from build123d import *

# Parameters (mm, degrees)
SKETCH2_W           = 16.5
SKETCH2_H           = 15.758588826
BOSS_EXTRUDE1_DEPTH = 3
SKETCH3_W           = 16.5
SKETCH3_H           = 4.058588826
BOSS_EXTRUDE2_DEPTH = 1.4
SKETCH4_W           = 16.5
SKETCH4_H           = 10.7
SKETCH4_R           = 1.65
BOSS_EXTRUDE3_DEPTH = 3
SKETCH5_R           = 1.4
CUT_EXTRUDE1_DEPTH  = 3
CHAMFER1_SIZE       = 2
SKETCH6_R           = 4.45
CUT_EXTRUDE2_DEPTH  = 17


with BuildPart() as part:
    # Sketch2 → Boss-Extrude1 (new body)
    with BuildSketch(Plane.XY):
        with Locations((0, 3.620705587)):
            Rectangle(SKETCH2_W, SKETCH2_H)
    extrude(amount=BOSS_EXTRUDE1_DEPTH)

    # Sketch3 → Boss-Extrude2 (add)
    with BuildSketch(Plane(origin=(0, 0, 0), x_dir=(-1, 0, 0), z_dir=(0, 0, -1))):
        with Locations((0, -2.229294413)):
            Rectangle(SKETCH3_W, SKETCH3_H)
    extrude(amount=BOSS_EXTRUDE2_DEPTH)

    # Sketch4 → Boss-Extrude3 (add)
    with BuildSketch(Plane(origin=(0, 0, -1.4), x_dir=(-1, 0, 0), z_dir=(0, 0, -1))):
        with Locations((0, -5.55)):
            Rectangle(SKETCH4_W, SKETCH4_H)
        with Locations((-5.25, -7.2)):
            Circle(SKETCH4_R, mode=Mode.SUBTRACT)
        with Locations((5.25, -7.2)):
            Circle(SKETCH4_R, mode=Mode.SUBTRACT)
    extrude(amount=BOSS_EXTRUDE3_DEPTH)

    # Sketch5 → Cut-Extrude1 (cut)
    with BuildSketch(Plane(origin=(0, 0, 0), x_dir=(-1, 0, 0), z_dir=(0, 0, -1))):
        with Locations((-5.25, 3.5)):
            Circle(SKETCH5_R)
        with Locations((5.25, 3.5)):
            Circle(SKETCH5_R)
    extrude(amount=-CUT_EXTRUDE1_DEPTH, mode=Mode.SUBTRACT)

    # Chamfer1
    chamfer1_edges = [part.edges().sort_by_distance(p)[0] for p in [
        (8.25, -10.9, -2.9),
        (-8.25, -10.9, -2.9),
        (-8.25, 11.5, 1.5),
        (8.25, 11.5, 1.5),
    ]]
    chamfer(chamfer1_edges, length=CHAMFER1_SIZE)

    # Sketch6 → Cut-Extrude2 (cut)
    with BuildSketch(Plane(origin=(0, -0.2, 0), x_dir=(1, 0, 0), z_dir=(0, 1, 0))):
        with Locations((0, 8.5)):
            Circle(SKETCH6_R)
    extrude(amount=-CUT_EXTRUDE2_DEPTH, mode=Mode.SUBTRACT)


solid = part.part
Work out the finished part from the listing and answer in its coordinate system (mm). A direction names the side the tool comes from. Give positions to 0.01 mm unless a question says otherwise; leave off trailing zeros. Loops run counter-clockwise (first coordinate to the right, second up) from the corner with the lowest first, then second, coordinate; pieces in that order, holes last. Notation, with made-up numbers: (35.25, -13) -> (66.25, -13) arc R24 ccw to (66.25, 26) -> close; hole circle Ø2 at (58, 89). An arc over 180 degrees is marked (long way). Use a Markdown table: item, result. Add a question column.
1) Which of the six approach directions +Z, -Z, +X, -X, +Y, -Y give full straight-line access (tool end or side, diameter ignored) to faces 1 (the flat face through (0, 6, 0)), 2 (the cylindrical face through (-4.034, -6.085, -2.879)), 3 (the flat face through (0, -4.259, 1))?
2) Consider line 1 along Y through (x, z) = (-5.25, 1.6); line 2 along X through (y, z) = (4.75, 1); line 3 along Y through (x, z) = (-5.25, -2.25). Determine where each line is inside the solid, lowest interval first.
3) The part is cut by section B-B, the plane z = -2.5. Determine the outline of the cut face in (x, y), plus the area to 3 significant figures.
4) The part is cut by section D-D, the plane x = -3. Determine the outline of the cut face in (y, z).
5) The part is cut by section C-C, the plane x = -5.25. Determine the outline of the cut face in (y, z), plus the area to 3 significant figures.
6) The part is cut by section A-A, the plane y = 3.5. Determine the outline of the cut face in (x, z).
7) Each of these flat-tipped pins is pushed along its axis until it touches: P1, Ø2, axis at x = -3.5, y = -7.5, coming from the +Z side; P2, Ø1, axis at x = 5, y = 6.5, coming from the -Z side; P3, Ø2, axis at x = -3.5, z = -3, coming from the +Y side. Where does it stop, or does it pass through?
8) For a pull along Y with two mould halves and no side action, classify faces 4 (the flat face through (-8.25, 0.2, 0.2)), 5 (the flat face through (0, 11.5, 1)), 6 (the cylindrical face through (-5.9, 2.26, 1.48)) as +Y half, -Y half, draft (parallel to the pull), parting line (faces both ways), or undercut.
Reported:
| question | item | result |
|---|---|---|
| 1 | face 1 | -Z, +X, -X, +Y |
| 1 | face 2 | +Z, -Z |
| 1 | face 3 | +Z, +X, -X, -Y |
| 2 | line 1 | y = -4.26 to 2.1, 4.9 to 11.5 |
| 2 | line 2 | x = -8.25 to -5.88, -4.62 to 4.62, 5.88 to 8.25 |
| 2 | line 3 | y = -10.9 to -8.85, -5.55 to -0.2 |
| 3 | outline | (-8.25, -8.9) -> (-6.25, -10.9) -> (6.25, -10.9) -> (8.25, -8.9) -> (8.25, -0.2) -> (-8.25, -0.2) -> close; hole circle Ø3.3 at (-5.25, -7.2); hole circle Ø3.3 at (5.25, -7.2) |
| 3 | area | 155 mm^2 |
| 4 | outline | (-10.9, -4.4) -> (-0.2, -4.4) -> (-0.2, 0) -> (11.5, 0) -> (11.5, 3) -> (-4.26, 3) -> (-4.26, -1.4) -> (-10.9, -1.4) -> close |
| 5 | outline | (-10.9, -4.4) -> (-8.85, -4.4) -> (-8.85, -1.4) -> (-10.9, -1.4) -> close; (-5.55, -4.4) -> (-0.2, -4.4) -> (-0.2, 0) -> (2.1, 0) -> (2.1, 3) -> (-4.26, 3) -> (-4.26, -1.4) -> (-5.55, -1.4) -> close; (4.9, 0) -> (11.5, 0) -> (11.5, 3) -> (4.9, 3) -> close |
| 5 | area | 66.8 mm^2 |
| 6 | outline | (-8.25, 0) -> (-6.65, 0) -> (-6.65, 3) -> (-8.25, 3) -> close; (-3.85, 0) -> (3.85, 0) -> (3.85, 3) -> (-3.85, 3) -> close; (6.65, 0) -> (8.25, 0) -> (8.25, 3) -> (6.65, 3) -> close |
| 7 | P1 | stops at z = -1.4 |
| 7 | P2 | stops at z = 0 |
| 7 | P3 | stops at y = -0.2 |
| 8 | face 4 | draft |
| 8 | face 5 | +Y half |
| 8 | face 6 | undercut |
